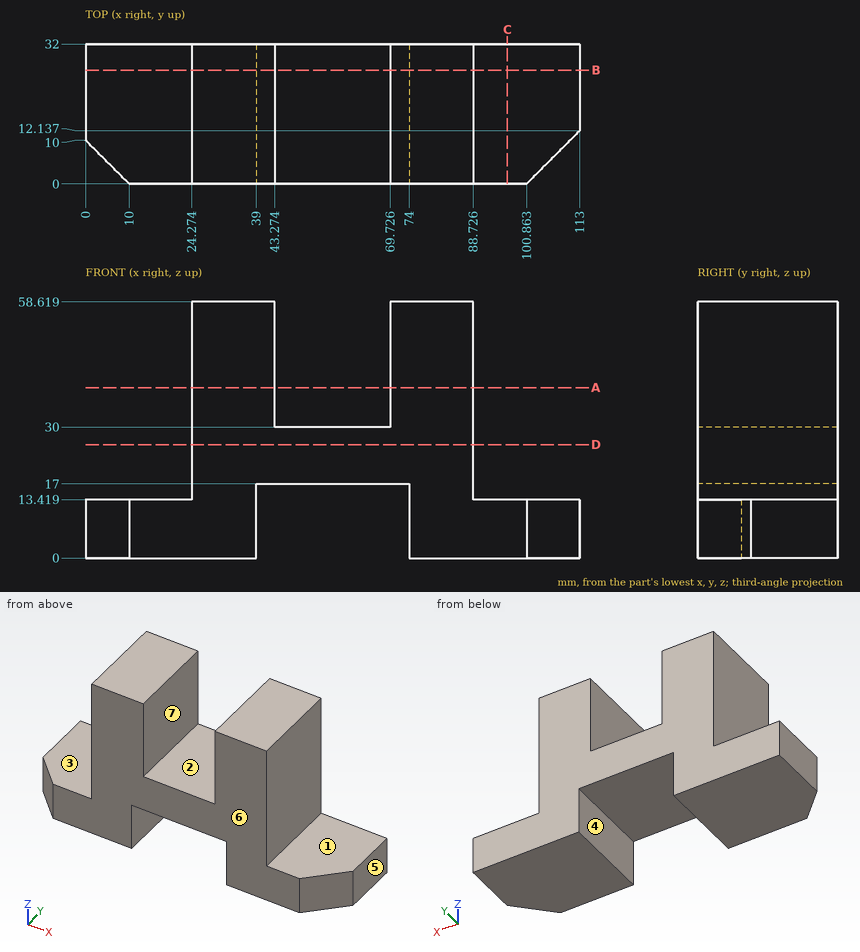
Could you check a few things on this drawing? It's one solid part, dimensions in mm from its lowest x, y, z. A direction names the side the tool comes from. Give positions to 0.01 mm unless a question says otherwise; leave off trailing zeros. Order: outer loops, then holes, each group sorted by start corner. A loop starts at its lowest first (then second) coordinate and runs counter-clockwise, first axis right, second up. Notation, with made-up numbers: (48, -10.75) - (57, -10.75) arc R26 cw to (57, 12.25) - close; hole circle Ø5 at (-1, 52.25). An arc over 180 degrees is marked (long way). Return JSON: item names as keys, results as strings. Group by question number.
Q1. Suppose I cut it at C-C, the plane x = 96.5. Please give me the cut outline in (y, z).
Q2. Will these pins go through, and if not, where does the flat tip stop? pin 1 Ø10 at (x, z) = (53, 48.5) entering from +Y; pin 2 Ø12 at (y, z) = (9.5, 35) entering from +X; pin 3 Ø5 at (x, z) = (72, 24) entering from -Y; pin 4 Ø12 at (x, y) = (97, 12) entering from +Z.
Q3. Suppose I cut it at D-D, the plane z = 26. Please give me the cut outline in (x, y).
Q4. Thinking about a two-plate mould opening in X: for the marked faces 5, 6 and 7, which applies, pulls with the +X half, pulls with the -X half, needs draft (parallel to the pull), parting line crosses it, or undercut?
Q5. Suppose I cut it at B-B, the plane y = 26. Please give me the cut outline in (x, z), and give its area (3 significant figures).
Q6. Which directions (+Z, -Z, +X, -X, +Y, -Y) give clear straight access to the entire face, cutting with the end or side of a thin tool? Please do the marked faces 1, 2, 3 and 4.
Q7. Suppose I cut it at A-A, the plane z = 39. Please give me the cut outline in (x, y).
Q8. Please list where these lines run through material, in increasing order: line 1 along X through (y, z) = (20.5, 39.5); line 2 along X through (y, z) = (26, 15.5); line 3 along Z through (x, y) = (92.5, 6.5). Write a range as [from, to].
Resolved:
{
 "1": {"outline": "(0, 0) - (32, 0) - (32, 13.42) - (0, 13.42) - close"},
 "2": {"pin 1": "passes through", "pin 2": "stops at x = 88.73", "pin 3": "stops at y = 0", "pin 4": "stops at z = 13.42"},
 "3": {"outline": "(24.27, 0) - (88.73, 0) - (88.73, 32) - (24.27, 32) - close"},
 "4": {"face 5": "pulls with the +X half", "face 6": "needs draft", "face 7": "undercut"},
 "5": {"outline": "(0, 0) - (39, 0) - (39, 17) - (74, 17) - (74, 0) - (113, 0) - (113, 13.42) - (88.73, 13.42) - (88.73, 58.62) - (69.73, 58.62) - (69.73, 30) - (43.27, 30) - (43.27, 58.62) - (24.27, 58.62) - (24.27, 13.42) - (0, 13.42) - close", "area": "3,080 mm2"},
 "6": {"face 1": "+Z, +X, +Y, -Y", "face 2": "+Z, +Y, -Y", "face 3": "+Z, -X, +Y, -Y", "face 4": "-Z, +Y, -Y"},
 "7": {"outline": "(24.27, 0) - (43.27, 0) - (43.27, 32) - (24.27, 32) - close; (69.73, 0) - (88.73, 0) - (88.73, 32) - (69.73, 32) - close"},
 "8": {"line 1": "x = [24.27, 43.27], [69.73, 88.73]", "line 2": "x = [24.27, 39], [74, 88.73]", "line 3": "z = [0, 13.42]"}
}
